Check sheet for the modelled part. Datum: model origin and axes. Units: mm. Face numbers are marked on the shaded views. A direction names the side the tool comes from. Coordinates: 2 decimals unless noted, no trailing zeros. Loops run counter-clockwise (first coordinate to the right, second up) from the corner with the lowest first, then second, coordinate; pieces in that order, holes last. Notation, with made-up numbers: M -10.5,50 L -4.5,50 A19 ccw -4.5,84 Z; hole C 80.5,23.5 d3. An arc over 180 degrees is marked long. Write each question's results on one line, items separated by ' | '. Start each with the question number.
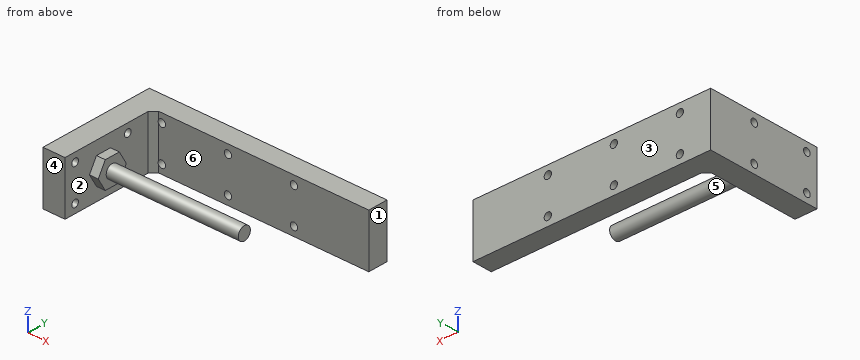
from build123d import *

# Parameters (mm, degrees)
BOSS_EXTRUDE1_DEPTH       = 24
CHAMFER1_SIZE             = 2.5
BOSS_EXTRUDE2_DEPTH       = 4
SKETCH3_R                 = 3
BOSS_EXTRUDE3_DEPTH       = 60
M4X0_7_TAPPED_HOLE1_D     = 3.3
M4X0_7_TAPPED_HOLE1_DEPTH = 10.1
M4X0_7_TAPPED_HOLE1_TIP   = 0.991420021
M4X0_7_TAPPED_HOLE2_D     = 3.3
M4X0_7_TAPPED_HOLE2_DEPTH = 10.1
M4X0_7_TAPPED_HOLE2_TIP   = 0.991420021


with BuildPart() as part:
    # Sketch1 → Boss-Extrude1 (new body)
    with BuildSketch(Plane.XY):
        Polygon((0, 0), (0, 52.5), (108, 52.5), (108, 43.5), (10, 43.5), (10, 0), align=None)
    extrude(amount=BOSS_EXTRUDE1_DEPTH)

    # Chamfer1
    chamfer1_edges = [part.edges().sort_by_distance(p)[0] for p in [
        (10, 43.5, 12),
    ]]
    chamfer(chamfer1_edges, length=CHAMFER1_SIZE)

    # Sketch2 → Boss-Extrude2 (add)
    with BuildSketch(Plane(origin=(10, 0, 0), x_dir=(0, 0, -1), z_dir=(1, 0, 0))):
        Polygon((-6, 22.464101615), (-12, 25.92820323), (-18, 22.464101615), (-18, 15.535898385), (-12, 12.07179677), (-6, 15.535898385), align=None)
    extrude(amount=BOSS_EXTRUDE2_DEPTH)

    # Sketch3 → Boss-Extrude3 (add)
    with BuildSketch(Plane(origin=(14, 0, 0), x_dir=(0, 0, -1), z_dir=(1, 0, 0))):
        with Locations(Location((-12, 19, 0), (0, 0, 90))):
            Circle(SKETCH3_R)
    extrude(amount=BOSS_EXTRUDE3_DEPTH)

    # M4x0.7 Tapped Hole1
    with Locations(Plane(origin=(0, 52.5, 0), x_dir=(1, 0, 0), z_dir=(0, 1, 0))):
        with Locations((14, -4), (44, -4), (74, -4), (74, -20), (44, -20), (14, -20)):
            Hole(M4X0_7_TAPPED_HOLE1_D / 2, depth=M4X0_7_TAPPED_HOLE1_DEPTH)
            with Locations((0, 0, -(M4X0_7_TAPPED_HOLE1_DEPTH + M4X0_7_TAPPED_HOLE1_TIP / 2))):  # 118° drill point
                Cone(0, M4X0_7_TAPPED_HOLE1_D / 2, M4X0_7_TAPPED_HOLE1_TIP, mode=Mode.SUBTRACT)

    # M4x0.7 Tapped Hole2
    with Locations(Plane.ZY):
        with Locations((4, 31), (20, 31), (20, 5), (4, 5)):
            Hole(M4X0_7_TAPPED_HOLE2_D / 2, depth=M4X0_7_TAPPED_HOLE2_DEPTH)
            with Locations((0, 0, -(M4X0_7_TAPPED_HOLE2_DEPTH + M4X0_7_TAPPED_HOLE2_TIP / 2))):  # 118° drill point
                Cone(0, M4X0_7_TAPPED_HOLE2_D / 2, M4X0_7_TAPPED_HOLE2_TIP, mode=Mode.SUBTRACT)


solid = part.part
Item 1: Tool access check on the marked faces 4, 5 and 6. Record the directions out of +Z, -Z, +X, -X, +Y, -Y that give a thin tool (end or side, any length) a straight path to the whole face; none if there is none.
Item 2: Section check C-C (y = 19). Record the cut outline in (x, z), plus the area to 3 significant figures.
Item 3: Thickness scan on line 1 (Z direction, x = 74, y = 46); line 2 (Y direction, x = 4.75, z = 20); line 3 (X direction, y = 46, z = 4). Record the ranges inside material, lowest first.
Item 4: Section check D-D (z = 10.5). Record the cut outline in (x, y).
Item 5: Release check for a two-part mould opening along Y. For the marked faces 1, 2 and 3 record: +Y half, -Y half, draft (parallel to the pull), parting line (faces both ways), or undercut.
Item 6: Section check B-B (y = 45). Record the cut outline in (x, z).
Item 7: Depth check by flat-ended pin: P1, Ø2, axis at x = 44, z = 20, coming from the -Y side; P2, Ø3, axis at x = 19, z = 8, coming from the -Y side; P3, Ø3, axis at y = 7, z = 9, coming from the -X side; P4, Ø13, axis at y = 19.5, z = 9, coming from the +X side. Enter the tip coordinate at first touch or a pass-through.
Item 8: Section check A-A (x = 44). Record the cut outline in (y, z).
Computed values:
1) face 4: +Z, -Z, +X, -X, -Y | face 5: +X | face 6: +Z, -Z, +X
2) outline: M 0,0 L 10,0 L 10,6 L 14,6 L 14,9 L 74,9 L 74,15 L 14,15 L 14,18 L 10,18 L 10,24 L 0,24 Z | area: 648 mm²
3) line 1: z = 0 to 2.35, 5.65 to 18.35, 21.65 to 24 | line 2: y = 0 to 3.35, 6.65 to 29.35, 32.65 to 52.5 | line 3: x = 0 to 12.35, 15.65 to 42.35, 45.65 to 72.35, 75.65 to 108
4) outline: M 0,0 L 10,0 L 10,12.94 L 14,12.94 L 14,16.4 L 74,16.4 L 74,21.6 L 14,21.6 L 14,25.06 L 10,25.06 L 10,41 L 12.5,43.5 L 108,43.5 L 108,52.5 L 0,52.5 Z
5) face 1: draft | face 2: undercut | face 3: +Y half
6) outline: M 0,0 L 108,0 L 108,24 L 0,24 Z; hole C 14,4 d3.3; hole C 14,20 d3.3; hole C 44,4 d3.3; hole C 44,20 d3.3; hole C 74,4 d3.3; hole C 74,20 d3.3
7) P1: passes through | P2: stops at y = 17.34 | P3: stops at x = 0 | P4: stops at x = 74
8) outline: C 19,12 d6; M 43.5,0 L 52.5,0 L 52.5,2.35 L 43.5,2.35 Z; M 43.5,5.65 L 52.5,5.65 L 52.5,18.35 L 43.5,18.35 Z; M 43.5,21.65 L 52.5,21.65 L 52.5,24 L 43.5,24 Z
